Source: CAD feature listing. Evaluate the final solid. Frame: model axes, mm. Coordinates: 2 decimals unless noted, no trailing zeros. Order: outer loops, then holes, each group sorted by start corner. A loop starts at its lowest first (then second) coordinate and runs counter-clockwise, first axis right, second up.
```python
from build123d import *

# Parameters (mm, degrees)
REVOLVE_2_ANGLE     = 180
SKETCH_3_R          = 3
CUT_EXTRUDE_1_DEPTH = 10
SKETCH_4_W          = 6.7
SKETCH_4_H          = 7
CUT_EXTRUDE_2_DEPTH = 20


with BuildPart() as part:
    # 草图1 → 旋转2 (revolve)
    with BuildSketch(Plane(origin=(0, 0, 0), x_dir=(0, 0, -1), z_dir=(1, 0, 0))):
        with BuildLine():
            Line((-16, 0), (-15, 0))
            ThreePointArc((-15, 0), (0, 15), (15, 0))
            Line((15, 0), (16, 0))
            ThreePointArc((16, 0), (0, 16), (-16, 0))
        make_face()
    revolve(axis=Axis((0, 0, -15), (0, 0, -1)), revolution_arc=REVOLVE_2_ANGLE)

    # 草图3 → 切除-拉伸1 (cut)
    with BuildSketch(Plane(origin=(20.295894922, 0, 0), x_dir=(0, 0, -1), z_dir=(1, 0, 0))):
        with Locations(Location((0, 0, 0), (0, 0, 180))):
            Circle(SKETCH_3_R)
    extrude(amount=-CUT_EXTRUDE_1_DEPTH, mode=Mode.SUBTRACT)

    # 草图4 → 切除-拉伸2 (cut)
    with BuildSketch(Plane(origin=(0, 27.814479009, 0), x_dir=(1, 0, 0), z_dir=(0, 1, 0))):
        with Locations((3.35, 0)):
            Rectangle(SKETCH_4_W, SKETCH_4_H)
    extrude(amount=-CUT_EXTRUDE_2_DEPTH, mode=Mode.SUBTRACT)


solid = part.part
```
Q1. Section query A-A on y = 0. Output: boundary loops of the cut face in (x, z).
Solutions:
outline: (0, -16) arc R16 ccw to (15.72, -3) - (14.7, -3) arc R15 cw to (0, -15) - close; (0, 15) arc R15 cw to (14.7, 3) - (15.72, 3) arc R16 ccw to (0, 16) - close
Q2. Material intervals for line 1 along Y through (x, z) = (1, 12.5); line 2 along Y through (x, z) = (9.25, -3); line 3 along Z through (x, y) = (7.25, 6.5), sorted ascending.
Solutions:
line 1: y = -9.94 to -8.23, 8.23 to 9.94
line 2: y = -12.71 to -11.42, 11.42 to 12.71
line 3: z = -12.7 to -11.41, 11.41 to 12.7
Q3. Section query B-B on z = 0. Output: boundary loops of the cut face in (x, y), plus the area to 3 significant figures.
Solutions:
outline: (0, -16) arc R16 ccw to (15.72, -3) - (14.7, -3) arc R15 cw to (0, -15) - close; (6.7, 13.42) arc R15 cw to (14.7, 3) - (15.72, 3) arc R16 ccw to (6.7, 14.53) - close
area: 35.7 mm2
Q4. Section query C-C on x = 13. Output: boundary loops of the cut face in (y, z).
Solutions:
outline: circle Ø18.65 at (0, 0); hole circle Ø14.97 at (0, 0)
Q5. Pin query (flat end, axial travel): P1, Ø3.5, axis at y = 0, z = 0, coming from the -X side; P2, Ø2, axis at x = 2, y = 13.5, coming from the -Z side; P3, Ø4, axis at x = 10, y = 9, coming from the +Z side; P4, Ø1.5, axis at y = 1, z = 9, coming from the -X side. Return the tip coordinate at first contact, or that it passes through.
Solutions:
P1: passes through
P2: stops at z = -9.8
P3: stops at z = 11.17
P4: stops at x = 11.35
Q6. Pull-direction query (Z, two-part tool) for faces 1 (the flat face through (0, -11, 11)), 2 (the flat face through (3, 15, 3.5)), 3 (the cylindrical face through (15.21, -0.9, 2.86)); classes: pulls with the +Z half, pulls with the -Z half, needs draft (parallel to the pull), parting line crosses it, or undercut.
Solutions:
face 1: needs draft
face 2: undercut
face 3: undercut
Q7. Section query D-D on y = 11.5. Output: boundary loops of the cut face in (x, z).
Solutions:
outline: (0, -11.12) arc R11.12 ccw to (0, 11.12) - (0, 9.63) arc R9.63 cw to (0, -9.63) - close
